Work out the finished part from the listing and answer in its coordinate system (mm). A direction names the side the tool comes from. Round coordinates to 2 decimals unless told otherwise and drop trailing zeros. Loops run counter-clockwise (first coordinate to the right, second up) from the corner with the lowest first, then second, coordinate; pieces in that order, holes last. Notation, with made-up numbers: (72.25, 80.25) -> (93.25, 80.25) arc R17 cw to (93.25, 93.25) -> close; hole circle Ø11 at (74.5, -30). An arc over 180 degrees is marked (long way). Use CSV: the item, a comma, the result in double quotes. Start each with the question number.
from build123d import *

# Parameters (mm, degrees)
F1_DEPTH = 3.175


with BuildPart() as f1:
    # F0 (on Top) → F1 (new body)
    with BuildSketch(Plane.XY):
        Polygon((-23.080186, 24.931203), (-48.480186, 24.931203), (-48.480186, 21.756203), (-51.655186, 21.756203), (-51.655186, 0.801203), (-48.480186, 0.801203), (-48.480186, -11.898797), (-51.655186, -11.898797), (-51.655186, -32.853797), (-48.480186, -32.853797), (-48.480186, -36.028797), (-23.080186, -36.028797), (-23.080186, -32.853797), (2.319814, -32.853797), (2.319814, -36.028797), (21.369814, -36.028797), (21.369814, -32.853797), (46.769814, -32.853797), (46.769814, -36.028797), (72.169814, -36.028797), (72.169814, -32.853797), (75.344814, -32.853797), (75.344814, -11.898797), (72.169814, -11.898797), (72.169814, 0.801203), (75.344814, 0.801203), (75.344814, 21.756203), (72.169814, 21.756203), (72.169814, 24.931203), (46.769814, 24.931203), (46.769814, 21.756203), (21.369814, 21.756203), (21.369814, 24.931203), (2.319814, 24.931203), (2.319814, 21.756203), (-23.080186, 21.756203), align=None)
    extrude(amount=-F1_DEPTH)


solid = f1.part
Q1. Section A-A, the plane x = 39 is taken. Write down the section's boundary in (y, z) (3 decimals), and give its area (3 significant figures).
Q2. Which of the six approach directions +Z, -Z, +X, -X, +Y, -Y give full straight-line access (tool end or side, diameter ignored) to faces 5 (the flat face through (-48.48, 23, -2)), 6 (the flat face through (-48.48, -34, -2)), 7 (the flat face through (-50, -11.899, -2))?
Q3. Each of these flat-tipped pins is pushed along its axis until it touches: pin 1 (6 mm diameter, centred on x = -21.5, y = -20.5, fed in from +Z); pin 2 (1 mm diameter, centred on y = 23, z = -1, fed in from +X); pin 3 (1.6 mm diameter, centred on y = -35, z = -1, fed in from -X); pin 4 (1 mm diameter, centred on x = 33, z = -1, fed in from +Y). Where does it stop, or does it pass through?
Q4. Section B-B, the plane y = -6 is taken. Write down the section's boundary in (x, z) (3 decimals).
Q5. A straight line is drawn through the part: line 1 (Y direction, x = -8, z = -0.75). Find the intervals that lie inside material, in ascending order. Write a range as from..to.
Q6. For a pull along Y with two mould halves and no side action, classify faces 1 (the flat face through (74, -11.899, -2)), 2 (the flat face through (74, 0.801, -2)), 3 (the flat face through (2.32, -34, -2)), 4 (the flat face through (74, -32.854, -2)) as pulls with the +Y half, pulls with the -Y half, needs draft (parallel to the pull), parting line crosses it, or undercut.
Report:
1,outline,"(-32.854, -3.175) -> (21.756, -3.175) -> (21.756, 0) -> (-32.854, 0) -> close"
1,area,"173 mm²"
2,face 5,"+Z, -Z, -X, +Y"
2,face 6,"+Z, -Z, -X, -Y"
2,face 7,"+Z, -Z, -X"
3,pin 1,"stops at z = 0"
3,pin 2,"stops at x = 72.17"
3,pin 3,"stops at x = -48.48"
3,pin 4,"stops at y = 21.76"
4,outline,"(-48.48, -3.175) -> (72.17, -3.175) -> (72.17, 0) -> (-48.48, 0) -> close"
5,line 1,"y = -32.85..21.76"
6,face 1,"undercut"
6,face 2,"undercut"
6,face 3,"needs draft"
6,face 4,"pulls with the -Y half"
